Part model, mm, in its own coordinate system. Face numbers are marked on the shaded views. A direction names the side the tool comes from. Coordinates: 2 decimals unless noted, no trailing zeros. Write each loop counter-clockwise with the first axis right and the second up, starting at its lowest first coordinate (ties: lowest second). Pieces come first, ordered by that corner, then holes. Notation, with made-up numbers: (-3, 41.25) - (21, 41.25) arc R24 ccw to (21, 60.25) - close; hole circle Ø6 at (84, -24.5). An arc over 180 degrees is marked (long way). Use a Markdown table: item, result.
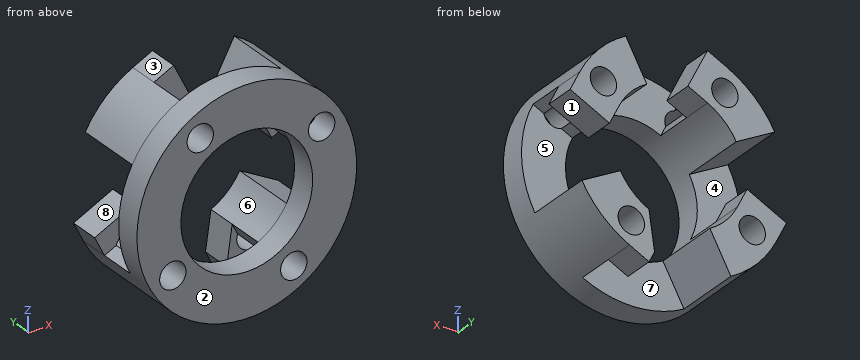
Autodesk Inventor part; units mm, degrees
ref_plane "YZ Plane" through (0, 0, 0) normal (1, 0, 0) x (0, 1, 0)
ref_plane "XZ Plane" through (0, 0, 0) normal (0, 1, 0) x (-1, 0, 0)
ref_plane "XY Plane" through (0, 0, 0) normal (0, 0, 1) x (1, 0, 0)
sketch "Sketch1" plane through (0, 0, 0) normal (0, 1, 0) x (-1, 0, 0)
  circle A0 centre (0, 0) radius 25
  circle A1 centre (0, 0) radius 15
  dimension "d0" = 50
  dimension "d1" = 30
extrude "Extrusion1" add sketch "Sketch1" along normal blind 6
sketch "Sketch2" plane through (0, 6, 0) normal (0, 1, 0) x (1, 0, 0)
  arc A0 (-6.6718, -13.4346) -> (-7.1782, 13.1709) centre (0, 0) ccw
  arc A1 (-21.9516, -11.9636) -> (-11.1196, -22.3909) centre (0, 0) ccw
  line L0 (-13.1709, -7.1782) -> (-21.9516, -11.9636)
  line L1 (-13.4346, 6.6718) -> (-22.3909, 11.1196)
  line L2 (-7.1782, 13.1709) -> (-11.9636, 21.9516)
  circle A2 centre (0, 0) radius 15
  line L3 (6.6718, 13.4346) -> (11.1196, 22.3909)
  circle A3 centre (0, 0) radius 25
  line L4 (13.1709, 7.1782) -> (21.9516, 11.9636)
  line L5 (-11.1196, -22.3909) -> (-6.6718, -13.4346)
  line L6 (7.1782, -13.1709) -> (11.9636, -21.9516)
  line L7 (13.4346, -6.6718) -> (22.3909, -11.1196)
  arc A4 (-22.3909, 11.1196) -> (-21.9516, -11.9636) centre (0, 0) ccw
  arc A5 (-11.1196, -22.3909) -> (21.9516, 11.9636) centre (0, 0) ccw
  arc A6 (-11.9636, 21.9516) -> (-22.3909, 11.1196) centre (0, 0) ccw
  arc A7 (11.1196, 22.3909) -> (-11.9636, 21.9516) centre (0, 0) ccw
  arc A8 (21.9516, 11.9636) -> (11.1196, 22.3909) centre (0, 0) ccw
  arc A9 (-13.1709, -7.1782) -> (-6.6718, -13.4346) centre (0, 0) ccw
  arc A10 (-13.4346, 6.6718) -> (-13.1709, -7.1782) centre (0, 0) ccw
  arc A11 (-7.1782, 13.1709) -> (-13.4346, 6.6718) centre (0, 0) ccw
  dimension "d6" = 35
  dimension "d7" = 35
  dimension "d8" = 35
  dimension "d9" = 35
  dimension "d10" = 55
  dimension "d11" = 55
  dimension "d12" = 55
  dimension "d13" = 55
extrude "Extrusion2" add sketch "Sketch2" along normal blind 15.5 contours L5 A1 L0 A2 | A0 L7 A3 L6 | L1 A3 L2 A2 | A0 L3 A3 L4
sketch "Sketch3" plane through (11.9636, 6, 21.9516) normal (-0.8781, 0, 0.4785) x (0.4785, 0, 0.8781)
  line L0 (-10, 15.5) -> (0, 15.5)
  line L1 (0, 15.5) -> (0, 9)
  line L2 (0, 9) -> (-10, 9)
  line L3 (-10, 9) -> (-10, 15.5)
  point P0 (-25, -6)
  dimension "d18" = 6.5
  dimension "d21" = 10
sketch "Sketch4" plane through (-21.9516, 6, 11.9636) normal (-0.4785, 0, -0.8781) x (-0.8781, 0, 0.4785)
  line L0 (0, 0) -> (0, 15.5)
  line L1 (-10, 15.5) -> (0, 15.5)
  line L2 (0, 15.5) -> (0, 9)
  line L3 (0, 9) -> (-10, 9)
  line L4 (-10, 9) -> (-10, 15.5)
  point P0 (-25, -6)
  dimension "d20" = 6.5
sketch "Sketch5" plane through (-11.9636, 6, -21.9516) normal (0.8781, 0, -0.4785) x (-0.4785, 0, -0.8781)
  line L0 (0, 0) -> (0, 15.5)
  line L1 (-10, 15.5) -> (0, 15.5)
  line L2 (0, 15.5) -> (0, 9)
  line L3 (0, 9) -> (-10, 9)
  line L4 (-10, 9) -> (-10, 15.5)
  point P0 (-25, -6)
  dimension "d19" = 6.5
sketch "Sketch6" plane through (21.9516, 6, -11.9636) normal (0.4785, 0, 0.8781) x (0.8781, 0, -0.4785)
  point P0 (-25, -6)
sketch "Sketch7" plane through (21.9516, 6, -11.9636) normal (0.4785, 0, 0.8781) x (0.8781, 0, -0.4785)
  line L0 (0, 0) -> (0, 15.5)
  line L1 (-10, 15.5) -> (0, 15.5)
  line L2 (0, 15.5) -> (0, 9)
  line L3 (0, 9) -> (-10, 9)
  line L4 (-10, 9) -> (-10, 15.5)
  point P0 (-25, -6)
  dimension "d17" = 6.5
sketch "Sketch12" plane through (-6.6718, 6, 13.4346) normal (0.8956, 0, 0.4448) x (0.4448, 0, -0.8956)
  line L0 (0, 0) -> (0, 15.5)
  line L1 (-10, 15.5) -> (0, 15.5)
  line L2 (0, 15.5) -> (0, 8.5)
  line L3 (0, 8.5) -> (-10, 8.5)
  line L4 (-10, 8.5) -> (-10, 15.5)
  point P0 (15, -6)
  dimension "d55" = 7
sketch "Sketch13" plane through (13.4346, 6, 6.6718) normal (0.4448, 0, -0.8956) x (-0.8956, 0, -0.4448)
  line L0 (0, 0) -> (0, 15.5)
  line L1 (-10, 15.5) -> (0, 15.5)
  line L2 (0, 15.5) -> (0, 8.5)
  line L3 (0, 8.5) -> (-10, 8.5)
  line L4 (-10, 8.5) -> (-10, 15.5)
  point P0 (15, -6)
  dimension "d56" = 7
sketch "Sketch14" plane through (6.6718, 6, -13.4346) normal (-0.8956, 0, -0.4448) x (-0.4448, 0, 0.8956)
  line L0 (-10, 15.5) -> (0, 15.5)
  line L1 (0, 15.5) -> (0, 8.5)
  line L2 (0, 8.5) -> (-10, 8.5)
  line L3 (-10, 8.5) -> (-10, 15.5)
  point P0 (15, -6)
  dimension "d57" = 7
sketch "Sketch15" plane through (-13.4346, 6, -6.6718) normal (-0.4448, 0, 0.8956) x (0.8956, 0, 0.4448)
  line L0 (0, 0) -> (0, 15.5)
  line L1 (-10, 15.5) -> (0, 15.5)
  line L2 (0, 15.5) -> (0, 8.5)
  line L3 (0, 8.5) -> (-10, 8.5)
  line L4 (-10, 8.5) -> (-10, 15.5)
  point P0 (15, -6)
  dimension "d58" = 7
extrude "Extrusion11" add sketch "Sketch12" along normal blind 5
extrude "Extrusion12" add sketch "Sketch13" along normal blind 5
sketch "Sketch16" plane through (6.6718, 6, -13.4346) normal (-0.8956, 0, -0.4448) x (-0.4448, 0, 0.8956)
  point P0 (15, -6)
extrude "Extrusion13" add sketch "Sketch14" along normal blind 5
extrude "Extrusion14" add sketch "Sketch15" along normal blind 5
sketch "Sketch8" plane through (0, 21.5, 0) normal (0, 1, 0) x (1, 0, 0)
  circle A0 centre (-16.8241, 10.5881) radius 3
  arc A1 (-7.1782, 13.1709) -> (-13.4346, 6.6718) centre (0, 0) ccw
  line L0 (-7.5733, 24.3443) -> (-2.7879, 15.5637)
  arc A2 (-11.9636, 21.9516) -> (-22.3909, 11.1196) centre (0, 0) ccw
  circle A3 centre (0, 0) radius 25
  line L1 (-22.3909, 11.1196) -> (-13.4346, 6.6718)
  line L2 (-15.6585, 2.1936) -> (-24.6149, 6.6414)
  line L3 (-16.8241, 10.5881) -> (-12.6951, 7.9896) construction
  dimension "d30" = 6
  dimension "d71" = 7
  dimension "d72" = 4.129
sketch "Sketch9" plane through (0, 21.5, 0) normal (0, 1, 0) x (1, 0, 0)
  circle A0 centre (10.6983, 17.046) radius 3
  line L0 (24.3443, 7.5733) -> (15.5637, 2.7879) construction
  arc A1 (21.9516, 11.9636) -> (11.1196, 22.3909) centre (0, 0) ccw construction
  line L1 (11.1196, 22.3909) -> (6.6718, 13.4346)
  line L2 (2.1936, 15.6585) -> (6.6414, 24.6149)
  line L3 (10.6983, 17.046) -> (13.2898, 21.175) construction
  dimension "d37" = 6
  dimension "d73" = 7
  dimension "d77" = 4.129
sketch "Sketch10" plane through (0, 21.5, 0) normal (0, 1, 0) x (1, 0, 0)
  circle A0 centre (17.046, -10.6983) radius 3
  line L0 (7.5733, -24.3443) -> (2.7879, -15.5637)
  arc A1 (11.9636, -21.9516) -> (22.3909, -11.1196) centre (0, 0) ccw construction
  line L1 (22.3909, -11.1196) -> (13.4346, -6.6718)
  line L2 (15.6585, -2.1936) -> (24.6149, -6.6414)
  line L3 (17.046, -10.6983) -> (21.175, -13.2898) construction
  dimension "d42" = 6
  dimension "d78" = 7
  dimension "d79" = 4.129
sketch "Sketch11" plane through (0, 21.5, 0) normal (0, 1, 0) x (1, 0, 0)
  circle A0 centre (-10.5881, -16.8241) radius 3
  line L0 (-24.3443, -7.5733) -> (-15.5637, -2.7879)
  arc A1 (-13.1709, -7.1782) -> (-6.6718, -13.4346) centre (0, 0) ccw construction
  line L1 (-11.1196, -22.3909) -> (-6.6718, -13.4346)
  line L2 (-2.1936, -15.6585) -> (-6.6414, -24.6149)
  line L3 (-10.5881, -16.8241) -> (-7.9896, -12.6951) construction
  dimension "d44" = 6
  dimension "d80" = 7
  dimension "d83" = 4.129
extrude "Extrusion15" cut sketch "Sketch8" against normal through all contours A0 L1 | L1 A0
extrude "Extrusion16" cut sketch "Sketch9" against normal through all
extrude "Extrusion17" cut sketch "Sketch10" against normal through all
extrude "Extrusion18" cut sketch "Sketch11" against normal through all
sketch "Sketch17" plane through (0, 21.5, 0) normal (0, 1, 0) x (1, 0, 0)
  line L0 (2.1936, 15.6585) -> (6.6414, 24.6149)
  line L1 (6.6718, 13.4346) -> (2.1936, 15.6585)
  line L2 (2.1936, 15.6585) -> (4.4175, 20.1367)
  line L3 (6.6718, 13.4346) -> (5.4119, 22.139)
  point P0 (0, 0)
extrude "Extrusion19" cut sketch "Sketch17" against normal blind 8
properties part number "male bayonet connector - mk2"
Item 1: Two-plate mould, pull along Z, no slides. Class the marked faces 1, 2 and 3: pulls with the +Z half, pulls with the -Z half, needs draft (parallel to the pull), parting line crosses it, or undercut.
From the geometry:
| item | result |
|---|---|
| face 1 | undercut |
| face 2 | needs draft |
| face 3 | pulls with the +Z half |
Item 2: Band-saw the part on D-D, the plane z = -6. Give the cut face in (x, y).
From the geometry:
| item | result |
|---|---|
| outline | (-24.27, 0) - (-13.75, 0) - (-13.75, 6) - (-24.27, 6) - close; (-23.32, 14.5) - (-13.77, 14.5) - (-13.77, 21.5) - (-23.32, 21.5) - close; (13.75, 0) - (24.27, 0) - (24.27, 6) - (13.75, 6) - close |
Item 3: Drop flat-ended pins along their axis: P1, Ø6, axis at x = 7, y = 4.5, coming from the -Z side; P2, Ø9.5, axis at x = -21, z = 2, coming from the +Y side; P3, Ø8, axis at y = 18.5, z = -8, coming from the -X side. Give the stop position or say it passes through.
From the geometry:
| item | result |
|---|---|
| P1 | z = -24.68 |
| P2 | y = 6 |
| P3 | x = -24.61 |
Item 4: Band-saw the part on B-B, the plane z = 0. Give the cut face in (x, y), then the cut area to 3 significant figures.
From the geometry:
| item | result |
|---|---|
| outline | (-25, 0) - (-15, 0) - (-15, 6) - (-25, 6) - close; (15, 0) - (25, 0) - (25, 6) - (15, 6) - close |
| area | 120 mm^2 |
Item 5: Band-saw the part on A-A, the plane x = 0. Give the cut face in (y, z).
From the geometry:
| item | result |
|---|---|
| outline | (0, -25) - (6, -25) - (6, -15) - (0, -15) - close; (0, 15) - (6, 15) - (6, 25) - (0, 25) - close |
Item 6: Which spindle directions (+Z, -Z, +X, -X, +Y, -Y) get a long thin tool onto all of the face, cutting with end or side? Do the marked faces 4, 5, 6, 7 and 8. Say none if no direction does.
From the geometry:
| item | result |
|---|---|
| face 4 | -X |
| face 5 | +X |
| face 6 | +Y, -Y |
| face 7 | -Z |
| face 8 | -X, +Y |
Item 7: Drill centre lines: probe 1 along Z at (x, y) = (-9, 15); probe 2 along X at (y, z) = (18, -10.5); probe 3 along Z at (x, y) = (10, 19.5). Where is each one in solid material? Low to high.
From the geometry:
| item | result |
|---|---|
| probe 1 | -16.51 to -12, 12 to 14.28, 19.37 to 23.44 |
| probe 2 | -22.7 to -19.82, -13.83 to -10.71, 10.71 to 19.27 |
| probe 3 | -22.95 to -19.96, -14.13 to -11.18, 11.18 to 18.35 |
Item 8: Band-saw the part on C-C, the plane y = 19. Count the separate pieces of the cut face and the enclosed holes in it, then the cut area to 4 significant figures.
From the geometry:
| item | result |
|---|---|
| separate pieces | 4 |
| enclosed holes | 4 |
| area | 557.5 mm^2 |
